from build123d import *

# Parameters (mm, degrees)
F0_R        = 6.35
F1_DEPTH    = 2.54
F2_R        = 0.9525
F3_DEPTH    = 3.81
F4_R        = 1.27
F5_DEPTH    = 12.7
F6_R        = 6.35
F7_DEPTH    = 3.81
F8_S5_R     = 0.9525
F8_T6_DEPTH = 11
F9_S5_R     = 1.27
F9_T6_DEPTH = 11


# Not quite as in the source:
# - a fillet or chamfer that OpenCascade refuses, or shapes differently, is made with other operations: its cross-section is extruded or revolved along the edge and cut away or added


with BuildPart() as f1:
    # F0 (on Top) → F1 (new body)
    with BuildSketch(Plane.XY):
        Circle(F0_R)
    extrude(amount=F1_DEPTH)

    # F2 (on face) → F3 (join)
    with BuildSketch(Plane.XY.offset(2.54)):
        Circle(F2_R)
    extrude(amount=F3_DEPTH)

    # F4 (on face) → F5 (join)
    with BuildSketch(Plane.XY.offset(6.35)):
        Circle(F4_R)
    extrude(amount=F5_DEPTH)

    # F6 (on face) → F7 (join)
    with BuildSketch(Plane.XY.offset(19.05)):
        Circle(F6_R)
    extrude(amount=F7_DEPTH)

    # F8: chamfer of 1.905 x 6.2309742382 on 1 edges, made by hand


with BuildPart() as f8_tool2:
    # F8_s3 → F8_t4 (revolve)
    with BuildSketch(Plane.XZ):
        Polygon((0.1190257618, 2.54), (6.35, 0.635), (6.35, 2.54), align=None)
    revolve(axis=Axis((0, 0, 2.54), (0, 0, 1)))

    # F8_s5 → F8_t6 (cut, symmetric)
    with BuildSketch(Plane.XY.offset(1.6)):
        Circle(F8_S5_R)
    extrude(amount=F8_T6_DEPTH, both=True, mode=Mode.SUBTRACT)


with BuildPart() as f1_1:
    add(f1.part)

    # F8_t1: cut F8_tool2
    add(f8_tool2.part, mode=Mode.SUBTRACT)

    # F9: chamfer of 1.905 x 6.2309742382 on 1 edges, made by hand


with BuildPart() as f9_tool2:
    # F9_s3 → F9_t4 (revolve)
    with BuildSketch(Plane.XZ):
        Polygon((6.35, 20.955), (0.1190257618, 19.05), (6.35, 19.05), align=None)
    revolve(axis=Axis((0, 0, 19.05), (0, 0, 1)))

    # F9_s5 → F9_t6 (cut, symmetric)
    with BuildSketch(Plane.XY.offset(20)):
        Circle(F9_S5_R)
    extrude(amount=F9_T6_DEPTH, both=True, mode=Mode.SUBTRACT)


with BuildPart() as f1_2:
    add(f1_1.part)

    # F9_t1: cut F9_tool2
    add(f9_tool2.part, mode=Mode.SUBTRACT)

    # F10: fillet of radius 6.35 on 1 edges, made by hand

    # F10_s1 → F10_t2 (revolve, cut)
    with BuildSketch(Plane.XZ):
        with BuildLine():
            ThreePointArc((6.35, 20.955), (4.2745373727, 22.3644107304), (1.8151929479, 22.86))
            Line((1.8151929479, 22.86), (6.35, 22.86))
            Line((6.35, 22.86), (6.35, 20.955))
        make_face()
    revolve(axis=Axis((0, 0, 22.86), (0, 0, 1)), mode=Mode.SUBTRACT)


solid = f1_2.part
CAD build for the part. Positions are in the model's coordinates, mm. A direction names the side the tool comes from. Coordinates: 2 decimals unless noted, no trailing zeros. Write each loop counter-clockwise with the first axis right and the second up, starting at its lowest first coordinate (ties: lowest second). Pieces come first, ordered by that corner, then holes. Notation, with made-up numbers: (24.5, -8.75) - (29.5, -8.75) arc R15 cw to (29.5, 18.25) - close; hole circle Ø11 at (75.5, 71.5). An arc over 180 degrees is marked (long way). Use a Markdown table: item, result. Add a question column.
Item 1: Band-saw the part on A-A, the plane z = 10.75. Give the cut face in (x, y).
Item 2: Drill centre lines: L1, parallel to Z at x = -1, y = 1.5; L2, parallel to Z at x = 4, y = -1.5; L3, parallel to Y at x = 0, z = 10. Where is each one in solid material? Low to high. Write a range as from..to.
Item 3: 3-axis set-ups, long thin cutter, end or side, ignore diameter. For faces 4 (the face through (-0.28, -1.26, 2.18)), 5 (the face through (0, 0, 22.86)): which of +Z, -Z, +X, -X, +Y, -Y reach the whole face in a straight line?
Item 4: Mould opens along Z. For faces 1 (the face through (-1.38, -6.2, 0.31)), 2 (the face through (0, 0, 0)), 3 (the face through (1.45, 0.46, 19.48)) say: pulls with the +Z half, pulls with the -Z half, needs draft (parallel to the pull), parting line crosses it, or undercut.
Item 5: Flat gauge pin, fed straight in: pin 1 (4 mm diameter, centred on y = 2.5, z = 10, fed in from -X). Where does the tip first touch, or does it go through?
Numbers:
| question | item | result |
|---|---|---|
| 1 | outline | circle Ø2.54 at (0, 0) |
| 2 | L1 | 0..2.03, 19.56..22.86 |
| 2 | L2 | 0..1.27, 20.32..22.37 |
| 2 | L3 | -1.27..1.27 |
| 3 | face 4 | none |
| 3 | face 5 | +Z, +X, -X, +Y, -Y |
| 4 | face 1 | needs draft |
| 4 | face 2 | pulls with the -Z half |
| 4 | face 3 | undercut |
| 5 | pin 1 | x = -1.17 |
